The listing builds one solid part. Answer for the finished solid, in the listing's coordinates (mm). Round coordinates to 2 decimals unless told otherwise and drop trailing zeros. Loops run counter-clockwise (first coordinate to the right, second up) from the corner with the lowest first, then second, coordinate; pieces in that order, holes last. Notation, with made-up numbers: (84.5, -21.75) -> (89.5, -21.75) arc R17 ccw to (89.5, -16.75) -> close; hole circle Ø4 at (45, -21.75). An arc over 180 degrees is marked (long way). Use a Markdown table: item, result. Add a question column.
Q1. Section A-A on z = -1.75 is taken. Give the number of separate pieces and of enclosed holes in the cut face, then the cut area to 3 significant figures.
Q2. Section C-C on x = -60.5 is taken. Give the vertices of the cut face in (y, z), then the cut area to 3 significant figures.
Q3. Section B-B on x = -25 is taken. Give the vertices of the cut face in (y, z), then the cut area to 3 significant figures.
Q4. Consider line 1 (Y direction, x = 25, z = -5.35); line 2 (Y direction, x = -50, z = -4.85); line 3 (Y direction, x = 0, z = -1.3). Determine where each line is inside the solid, lowest interval first.
Q5. Given pin 1 Ø4 at (x, y) = (-23, 59.5) entering from -Z; pin 2 Ø5 at (x, y) = (50, 35) entering from -Z; pin 3 Ø4 at (x, z) = (-67.5, -6) entering from +Y, each flat-ended and moving along its own axis, determine where each tip first touches the part or whether it passes through.
Q6. Section D-D on y = 44.5 is taken. Give the vertices of the cut face in (x, z).
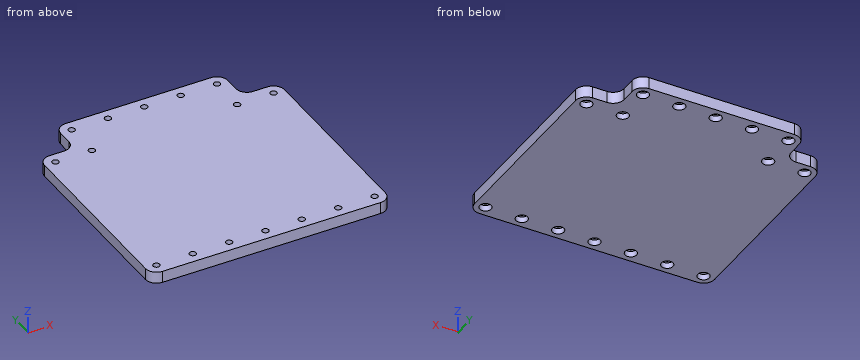
from build123d import *

# Parameters (mm, degrees)
BOSS_EXTRUDE1_DEPTH            = 8
CBORE_FOR_M4_SHCS1_D           = 4.5
CBORE_FOR_M4_SHCS1_CBORE_D     = 8
CBORE_FOR_M4_SHCS1_CBORE_DEPTH = 4


with BuildPart() as part:
    # Sketch2 → Boss-Extrude1 (new body)
    with BuildSketch(Plane.XY):
        with BuildLine():
            Line((-57.5, 60), (-57.5, 50))
            ThreePointArc((-57.5, 50), (-59.696699141, 44.696699141), (-65, 42.5))
            Line((-65, 42.5), (-75, 42.5))
            ThreePointArc((-75, 42.5), (-80.303300859, 40.303300859), (-82.5, 35))
            Line((-82.5, 35), (-82.5, -90))
            ThreePointArc((-82.5, -90), (-80.303300859, -95.303300859), (-75, -97.5))
            Line((-75, -97.5), (75, -97.5))
            ThreePointArc((75, -97.5), (80.303300859, -95.303300859), (82.5, -90))
            Line((82.5, -90), (82.5, 35))
            ThreePointArc((82.5, 35), (80.303300859, 40.303300859), (75, 42.5))
            Line((75, 42.5), (65, 42.5))
            ThreePointArc((65, 42.5), (59.696699141, 44.696699141), (57.5, 50))
            Line((57.5, 50), (57.5, 60))
            ThreePointArc((57.5, 60), (55.303300859, 65.303300859), (50, 67.5))
            Line((50, 67.5), (-50, 67.5))
            ThreePointArc((-50, 67.5), (-55.303300859, 65.303300859), (-57.5, 60))
        make_face()
    extrude(amount=-BOSS_EXTRUDE1_DEPTH)

    # CBORE for M4 SHCS1 (through all)
    with Locations(Plane(origin=(0, 0, -8), x_dir=(-1, 0, 0), z_dir=(0, 0, -1))):
        with Locations((-75, 35), (-50, 35), (-50, 60), (-25, 60), (0, 60), (25, 60), (50, 60), (50, 35), (75, 35), (-75, -90), (-50, -90), (-25, -90), (0, -90), (25, -90), (50, -90), (75, -90)):
            CounterBoreHole(CBORE_FOR_M4_SHCS1_D / 2, CBORE_FOR_M4_SHCS1_CBORE_D / 2, CBORE_FOR_M4_SHCS1_CBORE_DEPTH)


solid = part.part
Checked values:
| question | item | result |
|---|---|---|
| 1 | separate pieces | 1 |
| 1 | enclosed holes | 16 |
| 1 | area | 25,700 mm2 |
| 2 | outline | (-97.5, -8) -> (44, -8) -> (44, 0) -> (-97.5, 0) -> close |
| 2 | area | 1,130 mm2 |
| 3 | outline | (-97.5, -8) -> (-94, -8) -> (-94, -4) -> (-92.25, -4) -> (-92.25, 0) -> (-97.5, 0) -> close; (-87.75, -4) -> (-86, -4) -> (-86, -8) -> (56, -8) -> (56, -4) -> (57.75, -4) -> (57.75, 0) -> (-87.75, 0) -> close; (62.25, -4) -> (64, -4) -> (64, -8) -> (67.5, -8) -> (67.5, 0) -> (62.25, 0) -> close |
| 3 | area | 1,220 mm2 |
| 4 | line 1 | y = -97.5 to -94, -86 to 56, 64 to 67.5 |
| 4 | line 2 | y = -97.5 to -94, -86 to 31, 39 to 56, 64 to 67.5 |
| 4 | line 3 | y = -97.5 to -92.25, -87.75 to 57.75, 62.25 to 67.5 |
| 5 | pin 1 | stops at z = -8 |
| 5 | pin 2 | stops at z = -4 |
| 5 | pin 3 | stops at y = 42.5 |
| 6 | outline | (-59.9, -8) -> (59.9, -8) -> (59.9, 0) -> (-59.9, 0) -> close |
